The model under review builds one solid part; all positions refer to its coordinate system, in mm. Face numbers are marked on the shaded views. Round coordinates to 2 decimals unless told otherwise and drop trailing zeros. Write each loop counter-clockwise with the first axis right and the second up, starting at its lowest first coordinate (ties: lowest second). Pieces come first, ordered by that corner, then holes.
Item 1: Clearance check with flat-ended pins moving along their axes: pin 1 Ø2.5 at (x, z) = (-2, 1) entering from +Y; pin 2 Ø4 at (x, y) = (-3, 17.5) entering from +Z; pin 3 Ø1.5 at (x, y) = (3, 27) entering from -Z. State where each tip first meets the part, or that it passes through.
Item 2: Add section B-B (y = 2). Give the boundary of the cut face in (x, z).
Item 3: Draft analysis for pull direction Z (two halves, no side actions). For the marked faces 1, 2 and 3, state which applies: +Z half, -Z half, draft (parallel to the pull), parting line (faces both ways), or undercut.
Item 4: To check wall thickness, follow L1, parallel to X at y = 30.5, z = 0; L2, parallel to Y at x = -2.5, z = 3. State the ranges of each line that lie inside material, in increasing order.
Item 5: Add section A-A (x = 0). Give the boundary of the cut face in (y, z).
```python
from build123d import *

# Parameters (mm, degrees)
SKETCH1_R           = 6
BOSS_EXTRUDE1_DEPTH = 1
SKETCH2_R           = 6
SKETCH2_R_2         = 4.3
BOSS_EXTRUDE2_DEPTH = 37.86
CHAMFER1_SIZE       = 0.4


with BuildPart() as part:
    # Sketch1 → Boss-Extrude1 (new body)
    with BuildSketch(Plane(origin=(0, 0, 0), x_dir=(1, 0, 0), z_dir=(0, 1, 0))):
        Circle(SKETCH1_R)
    extrude(amount=BOSS_EXTRUDE1_DEPTH)

    # Sketch2 → Boss-Extrude2 (add)
    with BuildSketch(Plane(origin=(0, 1, 0), x_dir=(1, 0, 0), z_dir=(0, 1, 0))):
        Circle(SKETCH2_R)
        Circle(SKETCH2_R_2, mode=Mode.SUBTRACT)
    extrude(amount=BOSS_EXTRUDE2_DEPTH)

    # Chamfer1
    chamfer1_edges = [part.edges().sort_by_distance(p)[0] for p in [
        (-6, 0, 0),
    ]]
    chamfer(chamfer1_edges, length=CHAMFER1_SIZE)


solid = part.part
```
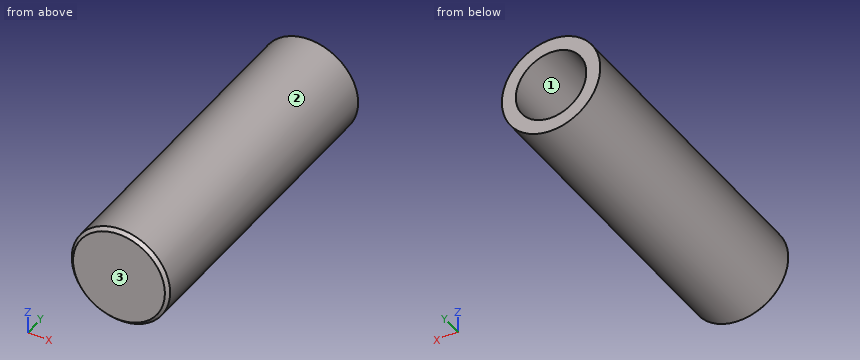
Numbers:
1. pin 1: stops at y = 1
1. pin 2: stops at z = 5.92
1. pin 3: stops at z = -5.56
2. outline: circle Ø12 at (0, 0); hole circle Ø8.6 at (0, 0)
3. face 1: undercut
3. face 2: parting line
3. face 3: draft
4. L1: x = -6 to -4.3, 4.3 to 6
4. L2: y = 0 to 1
5. outline: (0, -5.6) - (0.4, -6) - (38.86, -6) - (38.86, -4.3) - (1, -4.3) - (1, 4.3) - (38.86, 4.3) - (38.86, 6) - (0.4, 6) - (0, 5.6) - close
